For this review, use the dimensioned drawing (mm, ordinates from the lowest corner) and the shaded views. A direction names the side the tool comes from. Coordinates: 2 decimals unless noted, no trailing zeros. Write each loop counter-clockwise with the first axis right and the second up, starting at its lowest first coordinate (ties: lowest second). Pieces come first, ordered by that corner, then holes. Notation, with made-up numbers: M 20.5,84 L 60.5,84 A13 ccw 60.5,90 Z; hole C 36,-30 d6. An arc over 180 degrees is marked long. Return JSON: item names as keys, results as strings.
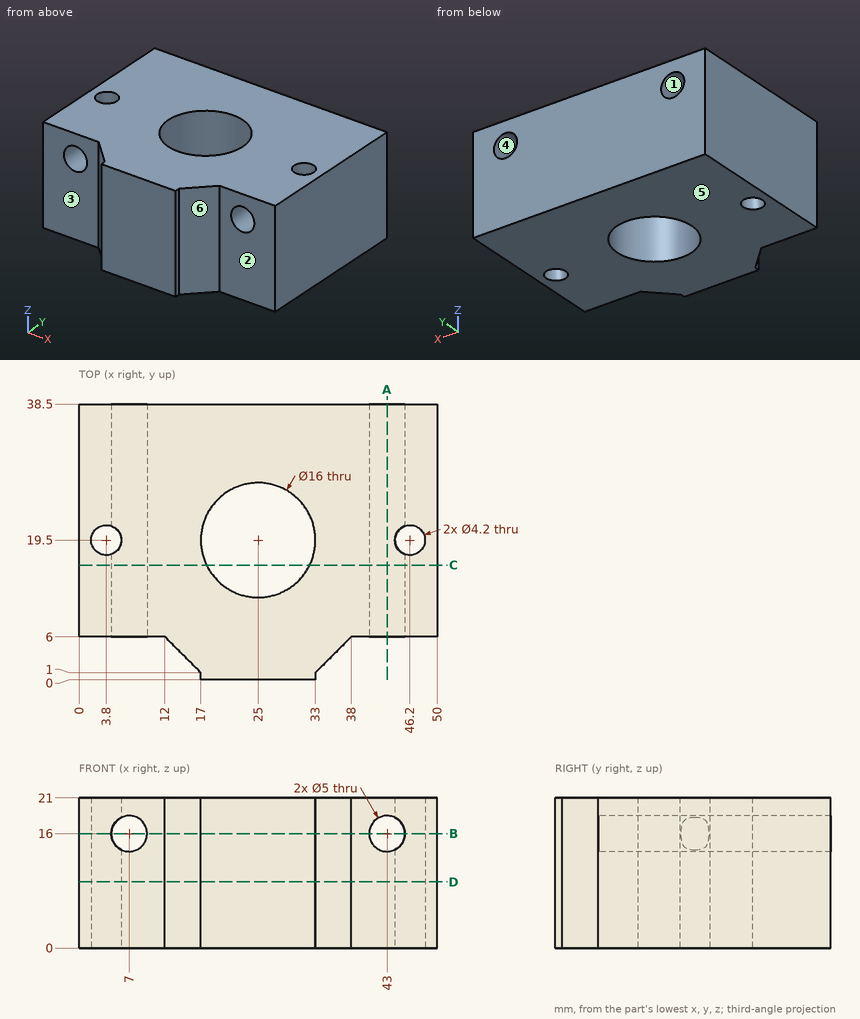
1. Wall thickness on L1, parallel to Y at x = 25, z = 12.75; L2, parallel to Z at x = 7, y = 21.5; L3, parallel to X at y = 8, z = 14.75: over which ranges is each line inside the solid? List them lowest first. Write a range as from..to.
Checks:
{"L1": "0..11.5, 27.5..38.5", "L2": "0..13.5, 18.5..21", "L3": "0..4.83, 9.17..40.83, 45.17..50"}
2. We need section D-D (z = 9.25). State the section outline as (x, y) points, plus the area to 3 significant figures.
Checks:
{"outline": "M 0,6 L 12,6 L 17,1 L 17,0 L 33,0 L 33,1 L 38,6 L 50,6 L 50,38.5 L 0,38.5 Z; hole C 3.8,19.5 d4.2; hole C 25,19.5 d16; hole C 46.2,19.5 d4.2", "area": "1,520 mm2"}
3. We need section C-C (y = 16). State the section outline as (x, z) points.
Checks:
{"outline": "M 0,0 L 17.81,0 L 17.81,21 L 0,21 Z; M 32.19,0 L 50,0 L 50,21 L 32.19,21 Z; hole C 7,16 d5; hole C 43,16 d5"}
4. Draft analysis for pull direction Z (two halves, no side actions). For the marked faces 4, 5 and 6, state which applies: +Z half, -Z half, draft (parallel to the pull), parting line (faces both ways), or undercut.
Checks:
{"face 4": "undercut", "face 5": "-Z half", "face 6": "draft"}
5. We need section B-B (z = 16). State the section outline as (x, y) points, plus the area to 3 significant figures.
Checks:
{"outline": "M 0,6 L 4.5,6 L 4.5,17.52 A2.1 cw long 4.5,21.48 L 4.5,38.5 L 0,38.5 Z; M 9.5,6 L 12,6 L 17,1 L 17,0 L 33,0 L 33,1 L 38,6 L 40.5,6 L 40.5,38.5 L 9.5,38.5 Z; M 45.5,6 L 50,6 L 50,38.5 L 45.5,38.5 L 45.5,21.48 A2.1 cw long 45.5,17.52 Z; hole C 25,19.5 d16", "area": "1,200 mm2"}
6. For the marked faces 1, 2 and 3, list the 3-axis set-ups (+Z, -Z, +X, -X, +Y, -Y) from which the entire face can be reached by the end or side of a thin tool; tool diameter is ignored.
Checks:
{"face 1": "+Y, -Y", "face 2": "+Z, -Z, +X, -Y", "face 3": "+Z, -Z, -X, -Y"}
7. We need section A-A (x = 43). State the section outline as (y, z) points, plus the area to 3 significant figures.
Checks:
{"outline": "M 6,0 L 38.5,0 L 38.5,13.5 L 6,13.5 Z; M 6,18.5 L 38.5,18.5 L 38.5,21 L 6,21 Z", "area": "520 mm2"}
8. Clearance check with flat-ended pins moving along their axes: pin 1 Ø9.5 at (x, z) = (43.5, 6) entering from -Y; pin 2 Ø1.1 at (y, z) = (0.5, 14) entering from +X; pin 3 Ø12 at (x, z) = (43.5, 11.5) entering from -Y. State where each tip first meets the part, or that it passes through.
Checks:
{"pin 1": "y = 6", "pin 2": "x = 33.05", "pin 3": "y = 5.5"}
